```python
from build123d import *

# Parameters (mm, degrees)
SKETCH2_W           = 42
SKETCH2_H           = 42
BOSS_EXTRUDE1_DEPTH = 42
SKETCH3_R           = 15.35
CUT_EXTRUDE2_DEPTH  = 5.4
SKETCH4_W           = 38.3
SKETCH4_H           = 38.3
CUT_EXTRUDE3_DEPTH  = 0.2
SKETCH5_R           = 15.35
CUT_EXTRUDE4_DEPTH  = 5.4
SKETCH6_W           = 38.3
SKETCH6_H           = 38.3
CUT_EXTRUDE5_DEPTH  = 0.2
SKETCH7_R           = 15.35
CUT_EXTRUDE6_DEPTH  = 5.4
SKETCH8_W           = 38.3
SKETCH8_H           = 38.3
CUT_EXTRUDE7_DEPTH  = 0.2
FILLET1_R           = 1.5


with BuildPart() as part:
    # Sketch2 → Boss-Extrude1 (new body)
    with BuildSketch(Plane.XY):
        Rectangle(SKETCH2_W, SKETCH2_H)
    extrude(amount=BOSS_EXTRUDE1_DEPTH)

    # Sketch3 → Cut-Extrude2 (cut)
    with BuildSketch(Plane(origin=(0, 21, 0), x_dir=(1, 0, 0), z_dir=(0, 1, 0))):
        with Locations(Location((0, -21, 0), (0, 0, 180))):
            Circle(SKETCH3_R)
    cut_extrude2 = extrude(amount=-CUT_EXTRUDE2_DEPTH, mode=Mode.SUBTRACT)

    # Sketch4 → Cut-Extrude3 (cut)
    with BuildSketch(Plane(origin=(0, 21, 0), x_dir=(1, 0, 0), z_dir=(0, 1, 0))):
        with Locations((0, -21)):
            Rectangle(SKETCH4_W, SKETCH4_H)
    cut_extrude3 = extrude(amount=-CUT_EXTRUDE3_DEPTH, mode=Mode.SUBTRACT)

    # Mirror1: Cut-Extrude2, Cut-Extrude3 across plane
    add(cut_extrude2.mirror(Plane.ZX), mode=Mode.SUBTRACT)
    add(cut_extrude3.mirror(Plane.ZX), mode=Mode.SUBTRACT)

    # Sketch5 → Cut-Extrude4 (cut)
    with BuildSketch(Plane(origin=(21, 0, 0), x_dir=(0, 0, -1), z_dir=(1, 0, 0))):
        with Locations(Location((-21, 0, 0), (0, 0, 90))):
            Circle(SKETCH5_R)
    cut_extrude4 = extrude(amount=-CUT_EXTRUDE4_DEPTH, mode=Mode.SUBTRACT)

    # Sketch6 → Cut-Extrude5 (cut)
    with BuildSketch(Plane(origin=(21, 0, 0), x_dir=(0, 0, -1), z_dir=(1, 0, 0))):
        with Locations((-21, 0)):
            Rectangle(SKETCH6_W, SKETCH6_H)
    cut_extrude5 = extrude(amount=-CUT_EXTRUDE5_DEPTH, mode=Mode.SUBTRACT)

    # Sketch7 → Cut-Extrude6 (cut)
    with BuildSketch(Plane.XY.offset(42)):
        Circle(SKETCH7_R)
    cut_extrude6 = extrude(amount=-CUT_EXTRUDE6_DEPTH, mode=Mode.SUBTRACT)

    # Sketch8 → Cut-Extrude7 (cut)
    with BuildSketch(Plane.XY.offset(42)):
        Rectangle(SKETCH8_W, SKETCH8_H)
    cut_extrude7 = extrude(amount=-CUT_EXTRUDE7_DEPTH, mode=Mode.SUBTRACT)

    # Mirror2: Cut-Extrude4, Cut-Extrude5 across plane
    add(cut_extrude4.mirror(Plane(origin=(0, 0, 0), x_dir=(0, 0, 1), z_dir=(1, 0, 0))), mode=Mode.SUBTRACT)
    add(cut_extrude5.mirror(Plane(origin=(0, 0, 0), x_dir=(0, 0, 1), z_dir=(1, 0, 0))), mode=Mode.SUBTRACT)

    # Mirror3: Cut-Extrude6, Cut-Extrude7 across plane
    add(cut_extrude6.mirror(Plane(origin=(0, 0, 21), x_dir=(1, 0, 0), z_dir=(0, 0, -1))), mode=Mode.SUBTRACT)
    add(cut_extrude7.mirror(Plane(origin=(0, 0, 21), x_dir=(1, 0, 0), z_dir=(0, 0, -1))), mode=Mode.SUBTRACT)

    # Fillet1
    fillet1_edges = [part.edges().sort_by_distance(p)[0] for p in [
        (21, 0, 42),
        (0, 21, 42),
        (-21, 0, 42),
        (0, 21, 0),
        (21, 0, 0),
        (0, -21, 0),
        (-21, 0, 0),
        (0, -21, 42),
        (-21, 21, 21),
        (21, 21, 21),
        (21, -21, 21),
        (-21, -21, 21),
    ]]
    fillet(fillet1_edges, radius=FILLET1_R)


solid = part.part
```
Design review of the part built by this model. Coordinates are the model's own, in mm. A direction names the side the tool comes from. Coordinates: 2 decimals unless noted, no trailing zeros. Answer in a Markdown table with one row per item.
(1) Wall thickness on line 1 along Z through (x, y) = (0, 17.4); line 2 along Y through (x, z) = (0, 39); line 3 along Y through (x, z) = (-19.6, 21): over which ranges is each line inside the solid? List them lowest first. Write a range as from..to.
Checked values:
| item | result |
|---|---|
| line 1 | 0.2..5.65, 36.35..41.8 |
| line 2 | -20.8..-15.35, 15.35..20.8 |
| line 3 | -21..-15.35, 15.35..21 |
(2) For faces 4 (the cylindrical face through (-7.08, -18.24, 7.38)), 5 (the cylindrical face through (18.24, -12.18, 11.66)), 6 (the flat face through (0, 0, 36.6)), list the 3-axis set-ups (+Z, -Z, +X, -X, +Y, -Y) from which the entire face can be reached by the end or side of a thin tool; tool diameter is ignored.
Checked values:
| item | result |
|---|---|
| face 4 | -Y |
| face 5 | +X |
| face 6 | +Z |
(3) Clearance check with flat-ended pins moving along their axes: pin 1 (15.5 mm diameter, centred on x = 6.5, z = 25, fed in from +Y); pin 2 (1 mm diameter, centred on y = 16.5, z = 6, fed in from +X); pin 3 (3 mm diameter, centred on x = 4, z = 8.5, fed in from +Y). State where each tip first meets the part, or that it passes through.
Checked values:
| item | result |
|---|---|
| pin 1 | y = 20.8 |
| pin 2 | x = 20.8 |
| pin 3 | y = 15.6 |
(4) The part is to be moulded in two halves that separate along Z. For faces 1 (the cylindrical face through (20.55, 0.27, 0.43)), 2 (the cylindrical face through (20.55, 0.27, 41.57)), 3 (the flat face through (-9, 20.8, 8)), say which applies: released by +Z, released by -Z, zero draft, split by the parting line, or undercut.
Checked values:
| item | result |
|---|---|
| face 1 | released by -Z |
| face 2 | released by +Z |
| face 3 | undercut |
